```python
from build123d import *

# Parameters (mm, degrees)
F0_R     = 1.25
F1_DEPTH = 7
F0_R_2   = 1
F2_DEPTH = 3
F3_DEPTH = 3
F4_DEPTH = 7
F0_W     = 6
F0_H     = 6
F0_W_2   = 22
F0_H_2   = 1
F5_DEPTH = 3
F0_W_3   = 38
F0_H_3   = 38
F6_DEPTH = 9
F7_DEPTH = 0.5
F8_DEPTH = 0.5


with BuildPart() as f1:
    # F0 (on Front) → F1 (new body)
    with BuildSketch(Plane.XZ):
        with BuildLine():
            ThreePointArc((-11.5, 14), (-11.7639320225, 15.1180339887), (-12.5, 16))
            ThreePointArc((-12.5, 16), (-15.767766953, 15.767766953), (-16, 12.5))
            ThreePointArc((-16, 12.5), (-13.209430585, 11.6282917549), (-11.5, 14))
        make_face()
        with Locations((-14, 14)):
            Circle(F0_R, mode=Mode.SUBTRACT)
    extrude(amount=F1_DEPTH)

    # F0 (on Front) → F4 (join)
    with BuildSketch(Plane.XZ):
        with BuildLine():
            Line((-11, 11), (-11, 16))
            Line((-11, 16), (-12.5, 16))
            ThreePointArc((-12.5, 16), (-11.7639320225, 15.1180339887), (-11.5, 14))
            ThreePointArc((-11.5, 14), (-13.209430585, 11.6282917549), (-16, 12.5))
            Line((-16, 12.5), (-16, 11))
            Line((-16, 11), (-11, 11))
        make_face()
        with BuildLine():
            Line((-11, 16), (-11, 17))
            Line((-11, 17), (-17, 17))
            Line((-17, 17), (-17, 11))
            Line((-17, 11), (-16, 11))
            Line((-16, 11), (-16, 12.5))
            ThreePointArc((-16, 12.5), (-15.767766953, 15.767766953), (-12.5, 16))
            Line((-12.5, 16), (-11, 16))
        make_face()
    extrude(amount=F4_DEPTH)



with BuildPart() as f1b:
    # F0 (on Front) → F1, piece 2 (new body)
    with BuildSketch(Plane.XZ):
        with BuildLine():
            ThreePointArc((12.5, 16), (12.232233047, 12.232233047), (16, 12.5))
            ThreePointArc((16, 12.5), (16.3717082451, 13.209430585), (16.5, 14))
            ThreePointArc((16.5, 14), (15.1180339887, 16.2360679775), (12.5, 16))
        make_face()
        with Locations((14, 14)):
            Circle(F0_R, mode=Mode.SUBTRACT)
    extrude(amount=F1_DEPTH)

    # F0 (on Front) → F4, piece 2 (join)
    with BuildSketch(Plane.XZ):
        with BuildLine():
            ThreePointArc((16.5, 14), (16.3717082451, 13.209430585), (16, 12.5))
            Line((16, 12.5), (16, 11))
            Line((16, 11), (17, 11))
            Line((17, 11), (17, 17))
            Line((17, 17), (11, 17))
            Line((11, 17), (11, 16))
            Line((11, 16), (12.5, 16))
            ThreePointArc((12.5, 16), (15.1180339887, 16.2360679775), (16.5, 14))
        make_face()
        with BuildLine():
            Line((16, 11), (16, 12.5))
            ThreePointArc((16, 12.5), (12.232233047, 12.232233047), (12.5, 16))
            Line((12.5, 16), (11, 16))
            Line((11, 16), (11, 11))
            Line((11, 11), (16, 11))
        make_face()
    extrude(amount=F4_DEPTH)


with BuildPart() as f1c:
    # F0 (on Front) → F1, piece 3 (new body)
    with BuildSketch(Plane.XZ):
        with BuildLine():
            ThreePointArc((-16, -12.5), (-15.767766953, -15.767766953), (-12.5, -16))
            ThreePointArc((-12.5, -16), (-11.7639320225, -15.1180339887), (-11.5, -14))
            ThreePointArc((-11.5, -14), (-13.209430585, -11.6282917549), (-16, -12.5))
        make_face()
        with Locations((-14, -14)):
            Circle(F0_R, mode=Mode.SUBTRACT)
    extrude(amount=F1_DEPTH)

    # F0 (on Front) → F4, piece 4 (join)
    with BuildSketch(Plane.XZ):
        with BuildLine():
            Line((-12.5, -16), (-11, -16))
            Line((-11, -16), (-11, -11))
            Line((-11, -11), (-16, -11))
            Line((-16, -11), (-16, -12.5))
            ThreePointArc((-16, -12.5), (-13.209430585, -11.6282917549), (-11.5, -14))
            ThreePointArc((-11.5, -14), (-11.7639320225, -15.1180339887), (-12.5, -16))
        make_face()
        with BuildLine():
            Line((-11, -17), (-11, -16))
            Line((-11, -16), (-12.5, -16))
            ThreePointArc((-12.5, -16), (-15.767766953, -15.767766953), (-16, -12.5))
            Line((-16, -12.5), (-16, -11))
            Line((-16, -11), (-17, -11))
            Line((-17, -11), (-17, -17))
            Line((-17, -17), (-11, -17))
        make_face()
    extrude(amount=F4_DEPTH)


with BuildPart() as f1d:
    # F0 (on Front) → F1, piece 4 (new body)
    with BuildSketch(Plane.XZ):
        with BuildLine():
            ThreePointArc((16.5, -14), (16.3717082451, -13.209430585), (16, -12.5))
            ThreePointArc((16, -12.5), (12.232233047, -12.232233047), (12.5, -16))
            ThreePointArc((12.5, -16), (15.1180339887, -16.2360679775), (16.5, -14))
        make_face()
        with Locations((14, -14)):
            Circle(F0_R, mode=Mode.SUBTRACT)
    extrude(amount=F1_DEPTH)

    # F0 (on Front) → F4, piece 3 (join)
    with BuildSketch(Plane.XZ):
        with BuildLine():
            Line((17, -11), (16, -11))
            Line((16, -11), (16, -12.5))
            ThreePointArc((16, -12.5), (16.3717082451, -13.209430585), (16.5, -14))
            ThreePointArc((16.5, -14), (15.1180339887, -16.2360679775), (12.5, -16))
            Line((12.5, -16), (11, -16))
            Line((11, -16), (11, -17))
            Line((11, -17), (17, -17))
            Line((17, -17), (17, -11))
        make_face()
        with BuildLine():
            Line((16, -12.5), (16, -11))
            Line((16, -11), (11, -11))
            Line((11, -11), (11, -16))
            Line((11, -16), (12.5, -16))
            ThreePointArc((12.5, -16), (12.232233047, -12.232233047), (16, -12.5))
        make_face()
    extrude(amount=F4_DEPTH)


with BuildPart() as f2:
    # F0 (on Front) → F2 (new body)
    with BuildSketch(Plane.XZ):
        with BuildLine():
            Line((-8.5, -2), (-8.5, 3.6e-09))
            Line((-8.5, 3.6e-09), (-8.5, 2))
            ThreePointArc((-8.5, 2), (-8.9750559736, 2.2802389662), (-9.5, 2.4494897428))
            ThreePointArc((-9.5, 2.4494897428), (-12.5, 0), (-9.5, -2.4494897428))
            ThreePointArc((-9.5, -2.4494897428), (-8.9750559736, -2.2802389662), (-8.5, -2))
        make_face()
        with Locations((-10, 0)):
            Circle(F0_R_2, mode=Mode.SUBTRACT)
    extrude(amount=F2_DEPTH)



with BuildPart() as f2b:
    # F0 (on Front) → F2, piece 2 (new body)
    with BuildSketch(Plane.XZ):
        with BuildLine():
            ThreePointArc((8.5, -1.9991173555), (12.4992939405, 0), (8.5, 1.9991173555))
            Line((8.5, 1.9991173555), (8.5, 0))
            Line((8.5, 0), (8.5, -1.9991173555))
        make_face()
        with Locations((10, 0)):
            Circle(F0_R_2, mode=Mode.SUBTRACT)
    extrude(amount=F2_DEPTH)


with BuildPart() as f2_1:
    add(f2.part)

    add(f2b.part)  # F3 merges F2b
    # F0 (on Front) → F3 (join)
    with BuildSketch(Plane.XZ):
        with BuildLine():
            Line((0, 8.5), (8.5, 8.5))
            Line((8.5, 8.5), (8.5, 1.9991173555))
            ThreePointArc((8.5, 1.9991173555), (12.4992939405, 0), (8.5, -1.9991173555))
            Line((8.5, -1.9991173555), (8.5, -8.5))
            Line((8.5, -8.5), (0, -8.5))
            Line((0, -8.5), (-8.5, -8.5))
            Line((-8.5, -8.5), (-8.5, -2))
            ThreePointArc((-8.5, -2), (-8.9750559736, -2.2802389662), (-9.5, -2.4494897428))
            Line((-9.5, -2.4494897428), (-9.5, -9.5))
            Line((-9.5, -9.5), (9.5, -9.5))
            Line((9.5, -9.5), (9.5, -2.4494897428))
            ThreePointArc((9.5, -2.4494897428), (12.5, 0), (9.5, 2.4494897428))
            Line((9.5, 2.4494897428), (9.5, 9.5))
            Line((9.5, 9.5), (-9.5, 9.5))
            Line((-9.5, 9.5), (-9.5, 2.4494897428))
            ThreePointArc((-9.5, 2.4494897428), (-8.9750559736, 2.2802389662), (-8.5, 2))
            Line((-8.5, 2), (-8.5, 8.5))
            Line((-8.5, 8.5), (0, 8.5))
        make_face()
    extrude(amount=F3_DEPTH)


with BuildPart() as f1_1:
    add(f1.part)

    add(f1b.part)  # F5 merges F1b

    add(f1c.part)  # F5 merges F1c

    add(f1d.part)  # F5 merges F1d

    add(f2_1.part)  # F5 merges F2
    # F0 (on Front) → F5 (join)
    with BuildSketch(Plane.XZ):
        Polygon((10, 16), (11, 16), (11, 17), (-11, 17), (-11, 16), (-10, 16), (0, 16), align=None)
        Polygon((16, 10.2088758318), (16, 11), (11, 11), (11, 16), (10, 16), (10, 10.2023985237), (10, 10), (0, 10), (0, 16), (-10, 16), (-11, 16), (-11, 11), (-16, 11), (-16, 10), (-10, 10), (-10, 4), (-16, 4), (-16, -11), (-11, -11), (-11, -16), (11, -16), (11, -11), (16, -11), align=None)
        with BuildLine():
            ThreePointArc((-9.5, -2.4494897428), (-12.5, 0), (-9.5, 2.4494897428))
            Line((-9.5, 2.4494897428), (-9.5, 9.5))
            Line((-9.5, 9.5), (9.5, 9.5))
            Line((9.5, 9.5), (9.5, 2.4494897428))
            ThreePointArc((9.5, 2.4494897428), (12.5, 0), (9.5, -2.4494897428))
            Line((9.5, -2.4494897428), (9.5, -9.5))
            Line((9.5, -9.5), (-9.5, -9.5))
            Line((-9.5, -9.5), (-9.5, -2.4494897428))
        make_face(mode=Mode.SUBTRACT)
        Polygon((10, 10.2023985237), (10, 16), (0, 16), (0, 10), (10, 10), align=None)
        with Locations((-13, 7)):
            Rectangle(F0_W, F0_H)
        Polygon((-16, 11), (-17, 11), (-17, -11), (-16, -11), (-16, 4), (-16, 10), align=None)
        with Locations((0, -16.5)):
            Rectangle(F0_W_2, F0_H_2)
        Polygon((17, 11), (16, 11), (16, 10.2088758318), (16, -11), (17, -11), align=None)
    extrude(amount=F5_DEPTH)

    # F0 (on Front) → F6 (join)
    with BuildSketch(Plane.XZ):
        Rectangle(F0_W_3, F0_H_3)
        Polygon((17, 17), (17, 11), (17, -11), (17, -17), (11, -17), (-11, -17), (-17, -17), (-17, -11), (-17, 11), (-17, 17), (-11, 17), (11, 17), align=None, mode=Mode.SUBTRACT)
    extrude(amount=F6_DEPTH)

    # F0 (on Front) → F7 (cut)
    with BuildSketch(Plane.XZ):
        with BuildLine():
            Line((-8.5, -2), (-8.5, 3.6e-09))
            Line((-8.5, 3.6e-09), (-8.5, 2))
            ThreePointArc((-8.5, 2), (-8.9750559736, 2.2802389662), (-9.5, 2.4494897428))
            ThreePointArc((-9.5, 2.4494897428), (-12.5, 0), (-9.5, -2.4494897428))
            ThreePointArc((-9.5, -2.4494897428), (-8.9750559736, -2.2802389662), (-8.5, -2))
        make_face()
        with Locations((-10, 0)):
            Circle(F0_R_2, mode=Mode.SUBTRACT)
    extrude(amount=F7_DEPTH, mode=Mode.SUBTRACT)

    # F0 (on Front) → F8 (cut)
    with BuildSketch(Plane.XZ):
        with BuildLine():
            ThreePointArc((8.5, -1.9991173555), (12.4992939405, 0), (8.5, 1.9991173555))
            Line((8.5, 1.9991173555), (8.5, 0))
            Line((8.5, 0), (8.5, -1.9991173555))
        make_face()
        with Locations((10, 0)):
            Circle(F0_R_2, mode=Mode.SUBTRACT)
    extrude(amount=F8_DEPTH, mode=Mode.SUBTRACT)


solid = f1_1.part
```
The listing builds one solid part. Answer for the finished solid, in the listing's coordinates (mm). A direction names the side the tool comes from. Give positions to 0.01 mm unless a question says otherwise; leave off trailing zeros. Order: outer loops, then holes, each group sorted by start corner. A loop starts at its lowest first (then second) coordinate and runs counter-clockwise, first axis right, second up. Notation, with made-up numbers: (15.25, -38) -> (69.25, -38) arc R7 cw to (69.25, -27) -> close; hole circle Ø1 at (-27, 38). An arc over 180 degrees is marked (long way). Answer as a JSON object with one key per item and string values. Group by question number.
Item 1: The part is cut by section D-D on x = -14. Write down the section's boundary in (y, z).
Item 2: The part is cut by section A-A on x = 7. Write down the section's boundary in (y, z), and give its area (3 significant figures).
Item 3: Consider L1, parallel to Z at x = -14, y = -4; L2, parallel to X at y = -7.5, z = 8; L3, parallel to X at y = -2.75, z = 5. Determine where each line is inside the solid, lowest interval first. Write a range as from..to.
Item 4: Determine the mould class of faces 6 (the flat face through (0, -4, 19)), 7 (the flat face through (-11, -5, -14)), 8 (the flat face through (0, 0, 9)) for opening direction Z: pulls with the +Z half, pulls with the -Z half, needs draft (parallel to the pull), parting line crosses it, or undercut.
Item 5: A tool of negligible diameter and unlimited length cuts with its end or side. For faces 1 (the flat face through (0, -4, -19)), 2 (the flat face through (11, -5, -14)), 3 (the flat face through (0, -1, 8.5)), 4 (the cylindrical face through (12.5, -0.25, -0.08)), 5 (the flat face through (-19, -4, 0)), from which of +Z, -Z, +X, -X, +Y, -Y can it reach the whole face along a straight path? Write none if from no direction.
Item 6: The part is cut by section B-B on y = -4.25. Write down the section's boundary in (x, z).
Item 7: Flat-ended cylindrical pins translate along their axes: pin 1 (3 mm diameter, centred on x = 14, z = -14, fed in from -Y); pin 2 (4 mm diameter, centred on x = 2, z = -8, fed in from +Y); pin 3 (5 mm diameter, centred on x = -4.5, z = 12, fed in from -Y). Find the tip coordinate at first contact, or state that the pin passes through.
Item 8: The part is cut by section C-C on z = 5.5. Write down the section's boundary in (x, y), and give its area (3 significant figures).
Result set:
{
 "1": {"outline": "(-9, -19) -> (0, -19) -> (0, -15.25) -> (-7, -15.25) -> (-7, -17) -> (-9, -17) -> close; (-9, 17) -> (-7, 17) -> (-7, 15.25) -> (0, 15.25) -> (0, 19) -> (-9, 19) -> close; (-7, -12.75) -> (0, -12.75) -> (0, 12.75) -> (-7, 12.75) -> (-7, 11) -> (-3, 11) -> (-3, -11) -> (-7, -11) -> close"},
 "2": {"outline": "(-9, -19) -> (0, -19) -> (0, -8.5) -> (-3, -8.5) -> (-3, -17) -> (-9, -17) -> close; (-9, 17) -> (-3, 17) -> (-3, 8.5) -> (0, 8.5) -> (0, 19) -> (-9, 19) -> close", "area": "87.0 mm²"},
 "3": {"L1": "-19..-15.25, -12.75..-11, 11..12.75, 15.25..19", "L2": "-19..-17, 17..19", "L3": "-19..-8.5, 8.5..19"},
 "4": {"face 6": "pulls with the +Z half", "face 7": "undercut", "face 8": "needs draft"},
 "5": {"face 1": "-Z, +X, -X, +Y, -Y", "face 2": "-Y", "face 3": "+Y, -Y", "face 4": "+Y", "face 5": "+Z, -Z, -X, +Y, -Y"},
 "6": {"outline": "(-19, -19) -> (19, -19) -> (19, 19) -> (-19, 19) -> close; hole (-17, -11) -> (-11, -11) -> (-11, -17) -> (11, -17) -> (11, -11) -> (17, -11) -> (17, 11) -> (11, 11) -> (11, 17) -> (-11, 17) -> (-11, 11) -> (-17, 11) -> close; hole circle Ø2.5 at (-14, -14); hole circle Ø2.5 at (-14, 14); hole circle Ø2.5 at (14, -14); hole circle Ø2.5 at (14, 14)"},
 "7": {"pin 1": "y = -7", "pin 2": "y = 0", "pin 3": "y = -3"},
 "8": {"outline": "(-19, -9) -> (-17, -9) -> (-17, -3) -> (-8.5, -3) -> (-8.5, 0) -> (-19, 0) -> close; (8.5, -3) -> (17, -3) -> (17, -9) -> (19, -9) -> (19, 0) -> (8.5, 0) -> close", "area": "87.0 mm²"}
}
